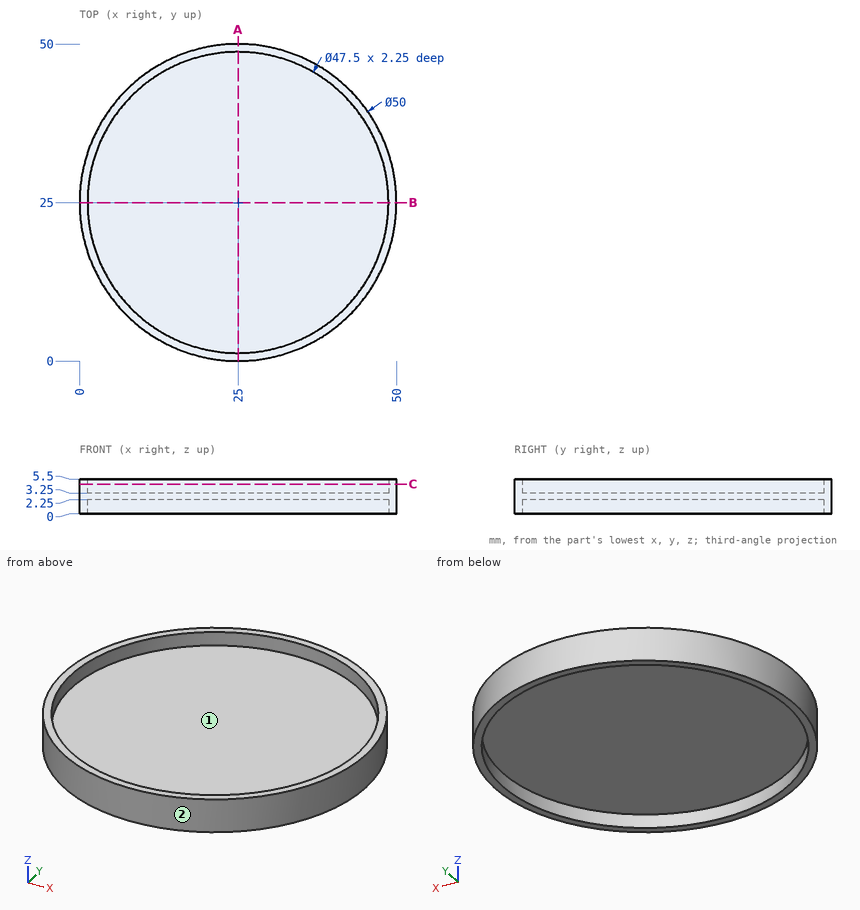
The figure shows three views and two pictorial views of one solid part (mm, origin at its lowest corner). Answer the questions. Coordinates: 2 decimals unless noted, no trailing zeros. Loops run counter-clockwise (first coordinate to the right, second up) from the corner with the lowest first, then second, coordinate; pieces in that order, holes last. Notation, with made-up numbers: (81, -4.5) - (97, -4.5) arc R14 ccw to (97, 0.5) - close; hole circle Ø2 at (75, 48). An arc over 180 degrees is marked (long way). Write item = value, one per line.
1) Determine the mould class of the marked faces 1 and 2 for opening direction Y: pulls with the +Y half, pulls with the -Y half, needs draft (parallel to the pull), parting line crosses it, or undercut.
Responses:
face_1 = undercut
face_2 = parting line crosses it
2) Section A-A (x = 25) is taken. Determine the outline of the cut face in (y, z).
Responses:
outline = (0, 0) - (1.25, 0) - (1.25, 2.25) - (48.75, 2.25) - (48.75, 0) - (50, 0) - (50, 5.5) - (48.75, 5.5) - (48.75, 3.25) - (1.25, 3.25) - (1.25, 5.5) - (0, 5.5) - close
3) Section C-C (z = 4.7) is taken. Determine the outline of the cut face in (x, y).
Responses:
outline = circle Ø50 at (25, 25); hole circle Ø47.5 at (25, 25)
4) Each of these flat-tipped pins is pushed along its axis until it touches: P1, Ø1, axis at x = 18.5, y = 21, coming from the +Z side; P2, Ø14, axis at x = 25.5, y = 27.5, coming from the -Z side; P3, Ø1.5, axis at x = 41.5, z = 2, coming from the +Y side. Where does it stop, or does it pass through?
Responses:
P1 = 3.25
P2 = 2.25
P3 = 44.41
5) Find the intervals of material crossed by line 1 along Y through (x, z) = (25, 4); line 2 along Y through (x, z) = (14, 4.1); line 3 along Z through (x, y) = (38, 42.5), in increasing order.
Responses:
line_1 = 0 to 1.25, 48.75 to 50
line_2 = 2.55 to 3.95, 46.05 to 47.45
line_3 = 2.25 to 3.25
